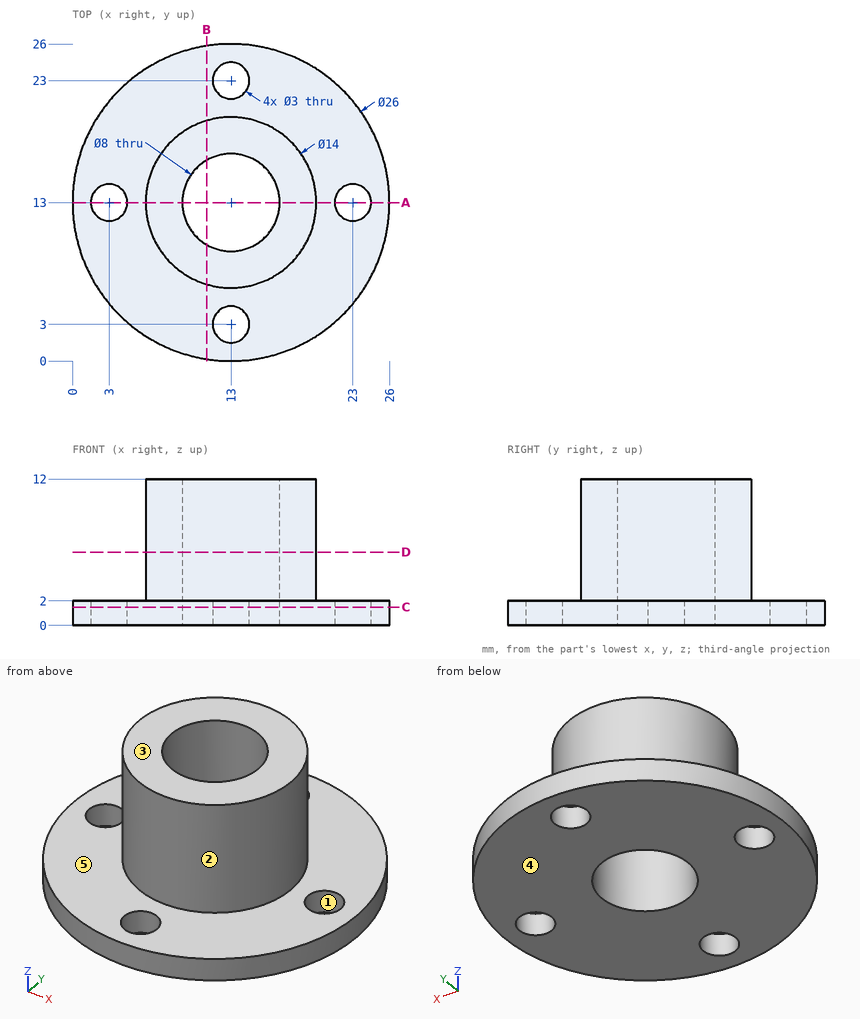
Job drawing, mm, ordinate dimensions from the low corner. One solid piece. A direction names the side the tool comes from. Give positions to 0.01 mm unless a question says otherwise; leave off trailing zeros. Loops run counter-clockwise (first coordinate to the right, second up) from the corner with the lowest first, then second, coordinate; pieces in that order, holes last. Notation, with made-up numbers: M 37.25,41 L 74.25,41 A11 ccw 74.25,60 Z; hole C 41,27.5 d9. An arc over 180 degrees is marked long. Put each result on its own line as item: value. Start each with the question number.
1) Saw through at A-A (y = 13). List the corners of the cut face in (x, z).
2) Saw through at C-C (z = 1.5). List the corners of the cut face in (x, y).
3) Saw through at D-D (z = 6). List the corners of the cut face in (x, y), then the cut area to 3 significant figures.
4) Saw through at B-B (x = 11). List the corners of the cut face in (y, z), then the cut area to 3 significant figures.
5) 3-axis set-ups, long thin cutter, end or side, ignore diameter. For the marked faces 4 and 5: which of +Z, -Z, +X, -X, +Y, -Y reach the whole face in a straight line?
6) Flat gauge pins, fed straight in: pin 1 (6 mm diameter, centred on x = 14, z = 3.5, fed in from -Y); pin 2 (5 mm diameter, centred on x = 11.5, z = 7.5, fed in from +Y); pin 3 (1 mm diameter, centred on y = 9.5, z = 9.5, fed in from +X); pin 4 (1.5 mm diameter, centred on x = 13.5, z = 7.5, fed in from -Y). Where does each tip first touch, or does it go through?
7) Pull direction X, two halves, no side cores. Call the marked faces 1, 2 and 3: +X half, -X half, draft (parallel to the pull), parting line (faces both ways), or undercut.
8) Probe probe 1 along Y at (x, z) = (13, 2.5); probe 2 along Z at (x, y) = (9, 5.25); probe 3 along X at (y, z) = (14.5, 6.75). List the from-to ranges inside material, lowest first.
Numbers:
1. outline: M 0,0 L 1.5,0 L 1.5,2 L 0,2 Z; M 4.5,0 L 9,0 L 9,12 L 6,12 L 6,2 L 4.5,2 Z; M 17,0 L 21.5,0 L 21.5,2 L 20,2 L 20,12 L 17,12 Z; M 24.5,0 L 26,0 L 26,2 L 24.5,2 Z
2. outline: C 13,13 d26; hole C 3,13 d3; hole C 13,13 d8; hole C 13,3 d3; hole C 13,23 d3; hole C 23,13 d3
3. outline: C 13,13 d14; hole C 13,13 d8
3. area: 104 mm^2
4. outline: M 0.15,0 L 9.54,0 L 9.54,12 L 6.29,12 L 6.29,2 L 0.15,2 Z; M 16.46,0 L 25.85,0 L 25.85,2 L 19.71,2 L 19.71,12 L 16.46,12 Z
4. area: 102 mm^2
5. face 4: -Z, +X, -X, +Y, -Y
5. face 5: +Z
6. pin 1: y = 0
6. pin 2: y = 20
6. pin 3: x = 19.32
6. pin 4: y = 6
7. face 1: undercut
7. face 2: parting line
7. face 3: draft
8. probe 1: 6 to 9, 17 to 20
8. probe 2: 0 to 2
8. probe 3: 6.16 to 9.29, 16.71 to 19.84
